For this review, take the finished solid that the model builds, in its own axes (mm). A direction names the side the tool comes from. Coordinates: 2 decimals unless noted, no trailing zeros. Loops run counter-clockwise (first coordinate to the right, second up) from the corner with the lowest first, then second, coordinate; pieces in that order, holes last. Notation, with made-up numbers: M 16,-29.75 L 22,-29.75 A29 cw 22,-0.75 Z; hole C 8,7 d5. An arc over 180 degrees is marked long. Write each question's results on one line, items separated by ' | '. Start each with the question number.
```python
from build123d import *

# Parameters (mm, degrees)
BOSS_EXTRUDE1_DEPTH = 63.5
CUT_EXTRUDE3_DEPTH  = 12.7
SKETCH3_W           = 12.7
SKETCH3_H           = 25.4
BOSS_EXTRUDE2_DEPTH = 12.7


with BuildPart() as part:
    # Sketch1 → Boss-Extrude1 (new body)
    with BuildSketch(Plane(origin=(0, 0, 0), x_dir=(1, 0, 0), z_dir=(0, 1, 0))):
        Polygon((0, 0), (25.4, 0), (25.4, -12.7), (-12.7, -12.7), (-12.7, 25.4), (25.4, 25.4), (25.4, 12.7), (0, 12.7), align=None)
    extrude(amount=BOSS_EXTRUDE1_DEPTH)

    # Sketch2 → Cut-Extrude3 (cut)
    with BuildSketch(Plane(origin=(0, 0, -25.4), x_dir=(-1, 0, 0), z_dir=(0, 0, -1))):
        Polygon((-25.4, 44.45), (-19.05, 44.45), (-19.05, 50.8), (-12.7, 50.8), (-12.7, 12.7), (-19.088668149, 12.7), (-19.088668149, 19.05), (-25.4, 19.05), align=None)
    extrude(amount=-CUT_EXTRUDE3_DEPTH, mode=Mode.SUBTRACT)

    # Sketch3 → Boss-Extrude2 (add)
    with BuildSketch(Plane(origin=(25.4, 0, 0), x_dir=(0, 0, -1), z_dir=(1, 0, 0))):
        with Locations((-6.35, 12.7)):
            Rectangle(SKETCH3_W, SKETCH3_H)
    extrude(amount=BOSS_EXTRUDE2_DEPTH)


solid = part.part
```
Q1. Take a section at A-A, the plane x = 7.5. Give the boundary of the cut face in (y, z).
Q2. The part is to be moulded in two halves that separate along X. For faces 4 (the face through (22, 44.45, -19)), 5 (the face through (19.05, 48, -19)), 6 (the face through (25.4, 54, -19)), say which applies: pulls with the +X half, pulls with the -X half, needs draft (parallel to the pull), parting line crosses it, or undercut.
Q3. To check wall thickness, follow line 1 along Z through (x, y) = (12.5, 54); line 2 along X through (y, z) = (55, 10); line 3 along Z through (x, y) = (33.5, 23). State the ranges of each line that lie inside material, in increasing order.
Q4. Take a section at C-C, the plane y = 8. Give the boundary of the cut face in (x, z).
Q5. Insertion check: P1, Ø14, axis at y = 42.5, z = 8.5, coming from the +X side; P2, Ø3, axis at x = -5.5, z = -9.5, coming from the -Y side; P3, Ø3, axis at x = 25, z = -2.5, coming from the +Y side; P4, Ø4, axis at y = 24.5, z = -17, coming from the +X side. Each pin has a flat end and moves straight along its axis. Give the tip position at first contact, or say it passes through.
Q6. Take a section at B-B, the plane x = 24.5. Give the boundary of the cut face in (y, z), then the cut area to 3 significant figures.
Q7. For faces 1 (the face through (10, 31, -12.7)), 2 (the face through (16, 50.8, -19)), 3 (the face through (25.4, 44, 6)), list the 3-axis set-ups (+Z, -Z, +X, -X, +Y, -Y) from which the entire face can be reached by the end or side of a thin tool; tool diameter is ignored.
Q8. Take a section at D-D, the plane z = 6. Give the boundary of the cut face in (x, y).
Results:
1) outline: M 0,-25.4 L 63.5,-25.4 L 63.5,-12.7 L 0,-12.7 Z; M 0,0 L 63.5,0 L 63.5,12.7 L 0,12.7 Z
2) face 4: needs draft | face 5: undercut | face 6: pulls with the +X half
3) line 1: -25.4 to -12.7, 0 to 12.7 | line 2: -12.7 to 25.4 | line 3: 0 to 12.7
4) outline: M -12.7,-25.4 L 25.4,-25.4 L 25.4,-12.7 L 0,-12.7 L 0,0 L 38.1,0 L 38.1,12.7 L -12.7,12.7 Z
5) P1: x = 25.4 | P2: y = 0 | P3: through | P4: x = 12.7
6) outline: M 0,-25.4 L 19.05,-25.4 L 19.05,-12.7 L 0,-12.7 Z; M 0,0 L 63.5,0 L 63.5,12.7 L 0,12.7 Z; M 44.45,-25.4 L 63.5,-25.4 L 63.5,-12.7 L 44.45,-12.7 Z | area: 1,290 mm^2
7) face 1: +X, +Y, -Y | face 2: -Z | face 3: +Z, -Z, +X, +Y
8) outline: M -12.7,0 L 38.1,0 L 38.1,25.4 L 25.4,25.4 L 25.4,63.5 L -12.7,63.5 Z
